Build history of the part. All positions in model axes, mm. A direction names the side the tool comes from. Give positions to 0.01 mm unless a question says otherwise; leave off trailing zeros. Write each loop counter-clockwise with the first axis right and the second up, starting at its lowest first coordinate (ties: lowest second). Pieces come first, ordered by that corner, then holes.
Autodesk Inventor part; units mm, degrees
ref_plane "YZ Plane" through (0, 0, 0) normal (1, 0, 0) x (0, 1, 0)
ref_plane "XZ Plane" through (0, 0, 0) normal (0, 1, 0) x (-1, 0, 0)
ref_plane "XY Plane" through (0, 0, 0) normal (0, 0, 1) x (1, 0, 0)
sketch "草圖1" plane through (0, 0, 0) normal (0, 1, 0) x (-1, 0, 0)
  line L0 (0, 5) -> (3, 5)
  line L1 (3, 5) -> (3, 8)
  line L2 (50.7, 5) -> (53.7, 5)
  line L3 (50.7, -5) -> (53.7, -5)
  line L4 (50.7, -5) -> (50.7, -8)
  line L5 (3, -5) -> (3, -8)
  line L6 (0, -5) -> (3, -5)
  line L7 (3, -8) -> (50.7, -8)
  line L8 (53.7, -5) -> (53.7, 5)
  line L9 (50.7, 8) -> (3, 8)
  line L10 (0, 5) -> (0, -5)
  line L11 (0, 0) -> (0, -38.3248)
  line L12 (50.7, 5) -> (50.7, 8)
  dimension "d1" = 10
  dimension "d2" = 3
  dimension "d3" = 3
  dimension "d8" = 53.7
extrude "擠出1" add sketch "草圖1" along normal blind 3
properties part number "beam" material "木材 (楓木)"
1. Drop flat-ended pins along their axis: pin 1 (0.9 mm diameter, centred on x = -1.5, y = 2, fed in from +Z); pin 2 (1.5 mm diameter, centred on y = 1, z = -7, fed in from -X); pin 3 (0.9 mm diameter, centred on y = 2, z = 6.5, fed in from +X). Give the stop position or say it passes through.
2. Saw through at A-A on y = 0.8. Give the cut face in (x, z).
3. 3-axis set-ups, long thin cutter, end or side, ignore diameter. For faces 1 (the face through (-1, 1, -5)), 2 (the face through (-50.7, 1, -6)), 3 (the face through (-1, 1, 5)): which of +Z, -Z, +X, -X, +Y, -Y reach the whole face in a straight line?
4. Drill centre line: line 1 along X through (y, z) = (2.3, 5.75). Where is it in solid material? Low to high.
5. Saw through at B-B on z = -6.75. Give the cut face in (x, y).
Outcome:
1. pin 1: stops at z = 5
1. pin 2: stops at x = -50.7
1. pin 3: stops at x = -3
2. outline: (-53.7, -5) - (-50.7, -5) - (-50.7, -8) - (-3, -8) - (-3, -5) - (0, -5) - (0, 5) - (-3, 5) - (-3, 8) - (-50.7, 8) - (-50.7, 5) - (-53.7, 5) - close
3. face 1: -Z, +X, +Y, -Y
3. face 2: -Z, -X, +Y, -Y
3. face 3: +Z, +X, +Y, -Y
4. line 1: x = -50.7 to -3
5. outline: (-50.7, 0) - (-3, 0) - (-3, 3) - (-50.7, 3) - close
